The model under review builds one solid part; all positions refer to its coordinate system, in mm. Coordinates: 2 decimals unless noted, no trailing zeros. Write each loop counter-clockwise with the first axis right and the second up, starting at its lowest first coordinate (ties: lowest second). Pieces come first, ordered by that corner, then holes. Notation, with made-up numbers: (76.25, 33) -> (93.25, 33) arc R16 ccw to (93.25, 53) -> close; hole circle Ø2 at (47, 23). An arc over 180 degrees is marked (long way). Write each question's results on one line, items separated by ' | '.
Autodesk Inventor part; units mm, degrees
ref_plane "YZ Plane" through (0, 0, 0) normal (1, 0, 0) x (0, 1, 0)
ref_plane "XZ Plane" through (0, 0, 0) normal (0, 1, 0) x (-1, 0, 0)
ref_plane "XY Plane" through (0, 0, 0) normal (0, 0, 1) x (1, 0, 0)
sketch "Sketch1" plane through (0, 0, 0) normal (0, 1, 0) x (-1, 0, 0)
  line L0 (7.6807, 7.7641) -> (-42.3193, 7.7641)
  line L1 (7.6807, 7.7641) -> (-1.1191, -9.2324)
  line L2 (-17.3193, 7.7641) -> (-17.3193, -12.946)
  line L3 (-42.3193, 7.7641) -> (-33.5196, -9.2324)
  line L4 (-17.3193, -5.8724) -> (0.6205, -5.8724)
  line L5 (-35.2592, -5.8724) -> (-17.3193, -5.8724)
  point P0 (0, 0)
  dimension "d0" = 50
extrude "Extrusion1" add sketch "Sketch1" along normal blind 0.6
ref_plane "Work Plane1" through (17.3193, 0, -40.5229) normal (-1, 0, 0) x (0, 1, 0)
sketch "Sketch2" plane through (17.3193, 0, -40.5229) normal (-1, 0, 0) x (0, 1, 0)
  line L0 (0, -48.2871) -> (0, -34.6505)
  line L1 (0, -34.6505) -> (0.6, -34.6505)
  line L2 (0.6, -48.2871) -> (0.6, -34.6505)
  line L3 (0, -48.2871) -> (0.6, -48.2871)
  line L4 (0.3, -48.2871) -> (0.6, -46.3953)
  line L5 (0.6, -34.6505) -> (0.6, -48.2871)
  line L6 (0.3, -48.2871) -> (0, -46.3953)
  line L7 (0, -34.6505) -> (0, -48.2871)
  point P0 (0, -40.5229)
extrude "Extrusion2" cut sketch "Sketch2" along normal mid plane 50 contours L0 L6 L3 | L4 L2 L3
sketch "Sketch3" plane through (0, 0.6, 0) normal (0, 1, 0) x (1, 0, 0)
  line L0 (-7.6807, -7.7641) -> (-6.7012, -5.8724)
  line L1 (42.3193, -7.7641) -> (-7.6807, -7.7641)
  line L2 (41.3399, -5.8724) -> (42.3193, -7.7641)
  line L3 (-6.7012, -5.8724) -> (41.3399, -5.8724)
  line L4 (-0.6205, 5.8724) -> (-6.7012, -5.8724)
  line L5 (-6.7012, -5.8724) -> (-7.6807, -5.8724)
  line L6 (-7.6807, -5.8724) -> (-7.6807, -5.0905)
  line L7 (-7.6807, -5.0905) -> (-6.7012, -5.0905)
  line L8 (-6.7012, -5.0905) -> (-6.7012, -5.8724)
  line L9 (-6.7012, -5.8724) -> (41.3399, -5.8724)
  line L10 (-7.6807, -5.0905) -> (-5.684, -5.0905)
  line L11 (-5.684, -5.0905) -> (-5.684, -5.8724)
  line L12 (-5.684, -5.8724) -> (-7.6807, -5.8724)
  line L13 (-7.6807, -5.8724) -> (-7.6807, -5.0905)
  point P0 (0, 0)
  point P1 (-6.2964, -5.0905)
extrude "Extrusion3" add sketch "Sketch3" against normal up to surface (0.6 mm away) contours L8 L10 L4 | L5 L6 L7 L8
properties part number "nóż"
Q1. Add section B-B (y = 0.4). Write out the cut boundary in (x, z).
Solution:
outline: (-7.68, 5.09) -> (-6.3, 5.09) -> (-0.62, -5.87) -> (35.26, -5.87) -> (41.99, 7.13) -> (-7.35, 7.13) -> (-6.7, 5.87) -> (-7.68, 5.87) -> close
Q2. Add section C-C (z = -1.5). Write out the cut boundary in (x, y).
Solution:
outline: (-2.88, 0) -> (37.52, 0) -> (37.52, 0.6) -> (-2.88, 0.6) -> close
Q3. For line 1 (X direction, y = 0.3, z = 4.5); line 2 (X direction, y = 0.3, z = -2.5); line 3 (Y direction, x = 26.5, z = 7), list the stretches that pass through material, from the lowest coordinate up. Write a range as from..to.
Solution:
line 1: -5.99..40.63 | line 2: -2.37..37.01 | line 3: 0.18..0.42
Q4. Add section D-D (z = 2). Write out the cut boundary in (x, y).
Solution:
outline: (-4.7, 0) -> (39.34, 0) -> (39.34, 0.6) -> (-4.7, 0.6) -> close
Q5. Draft analysis for pull direction Z (two halves, no side actions). For faces 1 (the flat face through (-3.5, 0.3, -0.31)), 2 (the flat face through (-7.09, 0.3, 6.62)), 3 (the flat face through (16, 0.6, 0)), 4 (the flat face through (17.67, 0.45, 6.83)), state which applies: pulls with the +Z half, pulls with the -Z half, needs draft (parallel to the pull), parting line crosses it, or undercut.
Solution:
face 1: pulls with the -Z half | face 2: undercut | face 3: needs draft | face 4: pulls with the +Z half
